Work out the finished part from the listing and answer in its coordinate system (mm). Round coordinates to 2 decimals unless told otherwise and drop trailing zeros. Order: outer loops, then holes, each group sorted by start corner. A loop starts at its lowest first (then second) coordinate and runs counter-clockwise, first axis right, second up. Notation, with made-up numbers: (89.5, 20) -> (108.5, 20) arc R16 ccw to (108.5, 30) -> close; hole circle Ø5 at (1.25, 56). An arc over 180 degrees is marked (long way). Use one line per item in the form item = value.
```python
from build123d import *

# Parameters (mm, degrees)
SKETCH1_W            = 30
SKETCH1_H            = 35
BOSS_EXTRUDE1_DEPTH  = 5
M3_CLEARANCE_HOLE1_D = 3.4
CHAMFER1_SIZE        = 3


with BuildPart() as part:
    # Sketch1 → Boss-Extrude1 (new body)
    with BuildSketch(Plane.XY):
        Rectangle(SKETCH1_W, SKETCH1_H)
    extrude(amount=BOSS_EXTRUDE1_DEPTH)

    # M3 Clearance Hole1 (through all)
    with Locations(Plane.XY.offset(5)):
        with Locations((7.5, -7.5), (-7.5, 7.5), (-7.5, -7.5), (7.5, 7.5)):
            Hole(M3_CLEARANCE_HOLE1_D / 2)

    # Chamfer1
    chamfer1_edges = [part.edges().sort_by_distance(p)[0] for p in [
        (15, -17.5, 2.5),
        (-15, -17.5, 2.5),
        (-15, 17.5, 2.5),
        (15, 17.5, 2.5),
    ]]
    chamfer(chamfer1_edges, length=CHAMFER1_SIZE)


solid = part.part
```
Item 1: The part is cut by section C-C, the plane z = 2.5. Give the vertices of the cut face in (x, y).
Findings:
outline = (-15, -14.5) -> (-12, -17.5) -> (12, -17.5) -> (15, -14.5) -> (15, 14.5) -> (12, 17.5) -> (-12, 17.5) -> (-15, 14.5) -> close; hole circle Ø3.4 at (-7.5, -7.5); hole circle Ø3.4 at (-7.5, 7.5); hole circle Ø3.4 at (7.5, -7.5); hole circle Ø3.4 at (7.5, 7.5)
Item 2: A flat-ended cylindrical pin translates along its axis: P1, Ø2.5, axis at x = -7.5, y = -7.5, coming from the -Z side. Find the tip coordinate at first contact, or state that the pin passes through.
Findings:
P1 = through
Item 3: Determine the mould class of faces 1 (the cylindrical face through (-7.13, 5.84, 2.46)), 2 (the flat face through (13.5, 16, 2.5)), 3 (the flat face through (0, 17.5, 2)) for opening direction X: released by +X, released by -X, zero draft, split by the parting line, or undercut.
Findings:
face_1 = undercut
face_2 = released by +X
face_3 = zero draft
Item 4: Consider line 1 along Y through (x, z) = (7.5, 2); line 2 along Y through (x, z) = (-8.25, 4.1); line 3 along X through (y, z) = (15, 2.45). Determine where each line is inside the solid, lowest interval first.
Findings:
line_1 = -17.5 to -9.2, -5.8 to 5.8, 9.2 to 17.5
line_2 = -17.5 to -9.03, -5.97 to 5.97, 9.03 to 17.5
line_3 = -14.5 to 14.5
Item 5: The part is cut by section B-B, the plane y = -7.5. Give the vertices of the cut face in (x, z), and give its area (3 significant figures).
Findings:
outline = (-15, 0) -> (-9.2, 0) -> (-9.2, 5) -> (-15, 5) -> close; (-5.8, 0) -> (5.8, 0) -> (5.8, 5) -> (-5.8, 5) -> close; (9.2, 0) -> (15, 0) -> (15, 5) -> (9.2, 5) -> close
area = 116 mm^2
Item 6: The part is cut by section A-A, the plane x = 7.5. Give the vertices of the cut face in (y, z), and give its area (3 significant figures).
Findings:
outline = (-17.5, 0) -> (-9.2, 0) -> (-9.2, 5) -> (-17.5, 5) -> close; (-5.8, 0) -> (5.8, 0) -> (5.8, 5) -> (-5.8, 5) -> close; (9.2, 0) -> (17.5, 0) -> (17.5, 5) -> (9.2, 5) -> close
area = 141 mm^2
Item 7: The part is cut by section D-D, the plane x = -12.75. Give the vertices of the cut face in (y, z), and give its area (4 significant figures).
Findings:
outline = (-16.75, 0) -> (16.75, 0) -> (16.75, 5) -> (-16.75, 5) -> close
area = 167.5 mm^2
